Verification items for the finished model (mm, model axes). Face numbers are marked on the shaded views. Coordinates: 2 decimals unless noted, no trailing zeros. Write item = value, one per line. Start each with the question number.
from build123d import *

# Parameters (mm, degrees)
SKETCH2_W           = 25
SKETCH2_H           = 3
BOSS_EXTRUDE1_DEPTH = 32
CIRPATTERN1_COUNT   = 6
SKETCH5_R           = 6
BOSS_EXTRUDE2_DEPTH = 32
SKETCH6_R           = 3
AXLEHOLE_DEPTH      = 53.191951405
FILLET1_R           = 2


with BuildPart() as part:
    # Sketch1 → Revolve1 (revolve)
    with BuildSketch(Plane.XZ, mode=Mode.PRIVATE) as revolve1_sk:
        with BuildLine():
            Line((25, 0), (28, 0))
            Line((28, 0), (28, 1.5))
            Line((28, 1.5), (26.8, 1.5))
            Line((26.8, 1.5), (26.8, 4.5))
            Line((26.8, 4.5), (28, 4.5))
            Line((28, 4.5), (28, 6))
            Line((28, 6), (26.8, 6))
            Line((26.8, 6), (26.8, 28))
            Line((26.8, 28), (28, 28))
            Line((28, 28), (28, 29.5))
            Line((28, 29.5), (26.8, 29.5))
            Line((26.8, 29.5), (26.8, 32.5))
            Line((26.8, 32.5), (28, 32.5))
            Line((28, 32.5), (28, 33.999996833))
            Line((28, 33.999996833), (27, 33.999996833))
            ThreePointArc((27, 33.999996833), (25.585786438, 33.414213562), (25, 32))
            Line((25, 32), (25, 0))
        make_face()
    revolve(revolve1_sk.sketch.rotate(Axis((0, 0, 34), (0, 0, -1)), 180), axis=Axis((0, 0, 34), (0, 0, -1)))

    # Sketch2 → Boss-Extrude1 (add)
    with BuildSketch(Plane.XY):
        with Locations((12.5, 0)):
            Rectangle(SKETCH2_W, SKETCH2_H)
    boss_extrude1 = extrude(amount=BOSS_EXTRUDE1_DEPTH)

    # CirPattern1: Boss-Extrude1 ×6 about axis
    cirpattern1_axis = Axis((0, 0, 0), (0, 0, 1))
    for i in range(1, CIRPATTERN1_COUNT):
        add(boss_extrude1.rotate(cirpattern1_axis, i * 360 / CIRPATTERN1_COUNT))

    # Sketch5 → Boss-Extrude2 (add)
    with BuildSketch(Plane.XY):
        Circle(SKETCH5_R)
    extrude(amount=BOSS_EXTRUDE2_DEPTH)

    # Sketch6 → AxleHole (cut, through all)
    with BuildSketch(Plane.XY):
        with Locations(Location((0, 0, 0), (0, 0, 180))):
            Circle(SKETCH6_R)
    extrude(amount=AXLEHOLE_DEPTH, mode=Mode.SUBTRACT)

    # Fillet1
    # the kernel refuses this fillet: 2 mm, written as the material it adds along each edge
    with BuildSketch(Plane(origin=(-24.954959427, -1.5, 32), x_dir=(0.10620109039764976, -0.9943446728365121, 0), z_dir=(0, 0, -1))) as fillet1_piece_1:
        with BuildLine():
            CenterArc((2.224755634, -1.997850608), FILLET1_R, 87.343441845, 98.752929077)
            Line((0.236066288, -2.210252789), (0, 0))
            ThreePointArc((0, 0), (1.158726893, 0.026867397), (2.317453785, 0))
        make_face()
    extrude(amount=32)
    with BuildSketch(Plane(origin=(-13.776517819, -20.861628814, 32), x_dir=(-0.8080272015953212, 0.589145178612228, 0), z_dir=(0, 0, -1)), Plane(origin=(13.776517819, 20.861628814, 32), x_dir=(0.8080272015953204, -0.589145178612229, 0), z_dir=(0, 0, -1)), Plane(origin=(24.954959427, -1.5, 32), x_dir=(-0.10620109039765001, -0.994344672836512, 0), z_dir=(0, 0, -1)), Plane(origin=(-11.178441608, 22.361628814, 32), x_dir=(0.9142282919929711, 0.4051994942242834, 0), z_dir=(0, 0, -1)), Plane(origin=(-24.954959427, 1.5, 32), x_dir=(0.10620109039765026, 0.994344672836512, 0), z_dir=(0, 0, -1))) as fillet1_piece_2:
        with BuildLine():
            CenterArc((2.224755634, 1.997850608), FILLET1_R, 173.903629078, 98.752929077)
            Line((0.236066288, 2.210252789), (0, 0))
            ThreePointArc((0, 0), (1.158726893, -0.026867397), (2.317453785, 0))
        make_face()
    extrude(amount=32)
    with BuildSketch(Plane(origin=(-11.178441608, -22.361628814, 32), x_dir=(0.5000000000000002, 0.8660254037844387, 0), z_dir=(0, 0, -1)), Plane(origin=(13.776517819, -20.861628814, 32), x_dir=(-0.5000000000000002, 0.8660254037844387, 0), z_dir=(0, 0, -1)), Plane(origin=(24.954959427, 1.5, 32), x_dir=(-1, 0, 0), z_dir=(0, 0, -1)), Plane(origin=(11.178441608, 22.361628814, 32), x_dir=(-0.4999999999999994, -0.8660254037844389, 0), z_dir=(0, 0, -1)), Plane(origin=(-13.776517819, 20.861628814, 32), x_dir=(0.5000000000000007, -0.8660254037844382, 0), z_dir=(0, 0, -1))) as fillet1_piece_3:
        with BuildLine():
            CenterArc((2.222823584, 2), FILLET1_R, 171.247070923, 98.752929077)
            ThreePointArc((0.246116119, 2.304347826), (0.096342606, 1.15502726), (0, 0))
            Line((0, 0), (2.222823584, 0))
        make_face()
    extrude(amount=32)
    with BuildSketch(Plane(origin=(5.809475019, 1.5, 32), x_dir=(1, 0, 0), z_dir=(0, 0, -1)), Plane(origin=(4.203775615, -4.281152949, 32), x_dir=(0.5000000000000001, -0.8660254037844386, 0), z_dir=(0, 0, -1)), Plane(origin=(1.605699404, 5.781152949, 32), x_dir=(0.4999999999999986, 0.8660254037844394, 0), z_dir=(0, 0, -1)), Plane(origin=(-4.203775615, 4.281152949, 32), x_dir=(-0.5000000000000004, 0.8660254037844384, 0), z_dir=(0, 0, -1)), Plane(origin=(-5.809475019, -1.5, 32), x_dir=(-1, 0, 0), z_dir=(0, 0, -1)), Plane(origin=(-1.605699404, -5.781152949, 32), x_dir=(-0.4999999999999988, -0.8660254037844393, 0), z_dir=(0, 0, -1))) as fillet1_piece_4:
        with BuildLine():
            CenterArc((1.384272266, -2), FILLET1_R, 90, 64.055520228)
            ThreePointArc((-0.414164556, -1.125), (-0.178914596, -0.572869827), (0, 0))
            Line((0, 0), (1.384272266, 0))
        make_face()
    extrude(amount=32)
    with BuildSketch(Plane(origin=(4.203775615, 4.281152949, 32), x_dir=(0.6399622417657335, -0.7684063567632539, 0), z_dir=(0, 0, -1)), Plane(origin=(5.809475019, -1.5, 32), x_dir=(-0.3454783045035584, -0.9384267372135913, 0), z_dir=(0, 0, -1)), Plane(origin=(-1.605699404, 5.781152949, 32), x_dir=(0.9854405462692932, 0.1700203804503366, 0), z_dir=(0, 0, -1)), Plane(origin=(-5.809475019, 1.5, 32), x_dir=(0.3454783045035597, 0.9384267372135907, 0), z_dir=(0, 0, -1))) as fillet1_piece_5:
        with BuildLine():
            CenterArc((1.398617439, -1.989994715), FILLET1_R, 95.733483793, 64.055520228)
            Line((-0.478236035, -1.299038106), (0, 0))
            ThreePointArc((0, 0), (0.599407474, -0.030015856), (1.198814948, 0))
        make_face()
    extrude(amount=32)
    with BuildSketch(Plane(origin=(-4.203775615, -4.281152949, 32), x_dir=(-0.4999999999999996, -0.8660254037844388, 0), z_dir=(0, 0, -1))) as fillet1_piece_6:
        with BuildLine():
            CenterArc((1.384272266, 2), FILLET1_R, 205.944479772, 64.055520228)
            ThreePointArc((-0.414164556, 1.125), (-0.178914596, 0.572869827), (0, 0))
            Line((0, 0), (1.384272266, 0))
        make_face()
    extrude(amount=32)
    # the kernel refuses this fillet: 2 mm, written as the material it takes off along each edge
    with BuildSketch(Plane(origin=(-0.894300596, -1.45102593, 32), x_dir=(0.8660254037844385, 0.5000000000000003, 0), z_dir=(0.5000000000000003, -0.8660254037844386, 0))) as fillet1_2_piece_1_section:
        with BuildLine():
            CenterArc((FILLET1_R, -FILLET1_R), FILLET1_R, 90, 90)
            Line((0, -FILLET1_R), (0, 0))
            Line((0, 0), (FILLET1_R, 0))
        make_face()
    fillet1_2_piece_1 = extrude(amount=29.145484408, mode=Mode.PRIVATE)
    fillet1_2_piece_1 = fillet1_2_piece_1 & Plane(origin=(0, 0, 31.552739603), x_dir=(-1, 0, 0), z_dir=(0, 0, -1)) * Cylinder(25, 67, mode=Mode.PRIVATE)
    fillet1_2_piece_1 = fillet1_2_piece_1 - Plane(origin=(0, 0, 31.552739603), x_dir=(1, 0, 0), z_dir=(0, 0, -1)) * Cylinder(6, 67, mode=Mode.PRIVATE)
    add(fillet1_2_piece_1, mode=Mode.SUBTRACT)


solid = part.part
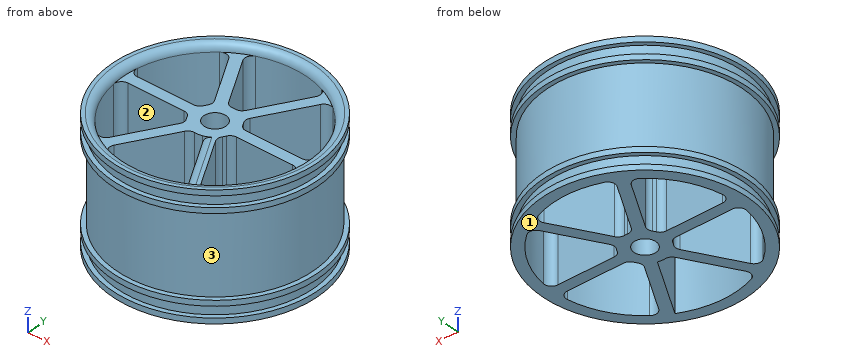
Item 1: Thickness scan on line 1 (Y direction, x = 0, z = 24); line 2 (X direction, y = -19, z = 2); line 3 (Y direction, x = 20, z = 13.5). Record the ranges inside material, lowest first.
Item 2: Gauge pin test, flat ends, axial feed: P1, Ø10, axis at x = -5.5, z = 20.5, coming from the +Y side; P2, Ø14, axis at x = 3, y = 6.5, coming from the +Z side; P3, Ø12.5, axis at x = -14.5, z = 17.5, coming from the -Y side. Record the tip position at first contact, or that the pin passes through.
Item 3: Mould release check, pull along X, two halves, no side actions. Record for the marked faces 1, 2 and 3: pulls with the +X half, pulls with the -X half, needs draft (parallel to the pull), parting line crosses it, or undercut.
Item 4: Section check A-A (x = -14.5). State how many separate pieces and enclosed holes the cut face has, then the cut area to 3 significant figures.
Filled sheet:
q1.line_1 = -26.8 to -25, -6 to -3, 3 to 6, 25 to 26.8
q1.line_2 = -18.9 to -16.25, -12.7 to -9.24, 9.24 to 12.7, 16.25 to 18.9
q1.line_3 = -17.84 to -15, -1.5 to 1.5, 15 to 17.84
q2.P1 = 26.8
q2.P2 = 32
q2.P3 = -25.5
q3.face_1 = needs draft
q3.face_2 = undercut
q3.face_3 = parting line crosses it
q4.separate_pieces = 3
q4.enclosed_holes = 0
q4.area = 286 mm^2
